Geometry: final body of the model. Coordinates: model frame, mm. Give positions to 0.01 mm unless a question says otherwise; leave off trailing zeros. Write each loop counter-clockwise with the first axis right and the second up, starting at its lowest first coordinate (ties: lowest second). Pieces come first, ordered by that corner, then holes. Notation, with made-up numbers: M 78.5,75.5 L 86.5,75.5 A25 ccw 86.5,105.5 Z; hole C -27.5,-9.5 d2. An arc over 180 degrees is marked long. Use a Markdown table: item, result. Add a question column.
(1) Cut plane C-C (y = 2.7). Output: boundary loops of the cut face in (x, z).
(2) Cut plane B-B (x = 0). Output: boundary loops of the cut face in (y, z), plus the area to 3 significant figures.
(3) Pin query (flat end, axial travel): pin 1 Ø4 at (x, z) = (-47, 0) entering from -Y; pin 2 Ø3 at (x, y) = (-22, 3) entering from +Z; pin 3 Ø1 at (y, z) = (0.5, -13) entering from -X; pin 4 Ø2 at (y, z) = (1, 10.5) entering from -X. Return the tip coordinate at first contact, or that it passes through.
(4) Material intervals for L1, parallel to X at y = 2.7, z = 0; L2, parallel to X at y = 4.55, z = 1.5; L3, parallel to X at y = 2.25, z = 35, sorted ascending.
(5) Cut plane D-D (x = 35.5). Output: boundary loops of the cut face in (y, z).
(6) Cut plane A-A (z = 0). Output: boundary loops of the cut face in (x, y).
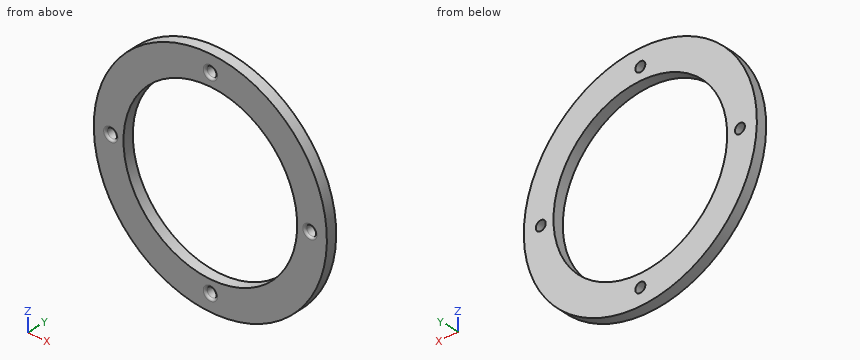
```python
from build123d import *

# Parameters (mm, degrees)
SKETCH_2_R          = 55
SKETCH_2_R_2        = 41
EXTRUDE_1_DEPTH     = 5
SKETCH_5_R          = 2.35
CUT_EXTRUDE_2_DEPTH = 5
FILLET_1_R          = 1


with BuildPart() as part:
    # 草图2 → 凸台-拉伸1 (new body)
    with BuildSketch(Plane(origin=(0, 0, 0), x_dir=(1, 0, 0), z_dir=(0, 1, 0))):
        with Locations(Location((0, 0, 0), (0, 0, 270))):
            Circle(SKETCH_2_R)
        with Locations(Location((0, 0, 0), (0, 0, 270))):
            Circle(SKETCH_2_R_2, mode=Mode.SUBTRACT)
    extrude(amount=EXTRUDE_1_DEPTH)

    # 草图5 → 切除-拉伸2 (cut)
    with BuildSketch(Plane(origin=(0, 0, 0), x_dir=(1, 0, 0), z_dir=(0, 1, 0))):
        with Locations(Location((0, -47, 0), (0, 0, 270))):
            Circle(SKETCH_5_R)
        with Locations(Location((-47, 0, 0), (0, 0, 270))):
            Circle(SKETCH_5_R)
        with Locations(Location((0, 47, 0), (0, 0, 270))):
            Circle(SKETCH_5_R)
        with Locations(Location((47, 0, 0), (0, 0, 270))):
            Circle(SKETCH_5_R)
    extrude(amount=CUT_EXTRUDE_2_DEPTH, mode=Mode.SUBTRACT)

    # 圆角1
    fillet_1_edges = [part.edges().sort_by_distance(p)[0] for p in [
        (0, 0, 44.65),
        (0, 0, -49.35),
        (-47, 0, -2.35),
        (47, 0, -2.35),
    ]]
    fillet(fillet_1_edges, radius=FILLET_1_R)


solid = part.part
```
Answer list:
| question | item | result |
|---|---|---|
| 1 | outline | C 0,0 d110; hole C -47,0 d4.7; hole C 0,0 d82; hole C 0,-47 d4.7; hole C 0,47 d4.7; hole C 47,0 d4.7 |
| 2 | outline | M 0,-55 L 5,-55 L 5,-49.35 L 1,-49.35 A1 ccw 0,-50.35 Z; M 0,-43.65 A1 ccw 1,-44.65 L 5,-44.65 L 5,-41 L 0,-41 Z; M 0,41 L 5,41 L 5,44.65 L 1,44.65 A1 ccw 0,43.65 Z; M 0,50.35 A1 ccw 1,49.35 L 5,49.35 L 5,55 L 0,55 Z |
| 2 | area | 92.1 mm² |
| 3 | pin 1 | through |
| 3 | pin 2 | z = 51.04 |
| 3 | pin 3 | x = -53.56 |
| 3 | pin 4 | x = -54.17 |
| 4 | L1 | -55 to -49.35, -44.65 to -41, 41 to 44.65, 49.35 to 55 |
| 4 | L2 | -54.98 to -48.81, -45.19 to -40.97, 40.97 to 45.19, 48.81 to 54.98 |
| 4 | L3 | -42.43 to -21.35, 21.35 to 42.43 |
| 5 | outline | M 0,-42.01 L 5,-42.01 L 5,-20.51 L 0,-20.51 Z; M 0,20.51 L 5,20.51 L 5,42.01 L 0,42.01 Z |
| 6 | outline | M -55,0 L -50.35,0 A1 ccw -49.35,1 L -49.35,5 L -55,5 Z; M -44.65,1 A1 ccw -43.65,0 L -41,0 L -41,5 L -44.65,5 Z; M 41,0 L 43.65,0 A1 ccw 44.65,1 L 44.65,5 L 41,5 Z; M 49.35,1 A1 ccw 50.35,0 L 55,0 L 55,5 L 49.35,5 Z |
